```python
from build123d import *

# Parameters (mm, degrees)
F0_R     = 7.5
F0_R_2   = 6
F1_DEPTH = 2
F2_R     = 0.5


# Not quite as in the source:
# - the program builds the solid bodies; features that only make, move or delete a surface that nothing else refers to are left out


with BuildPart() as f1:
    # F0 (on Front) → F1 (new body)
    with BuildSketch(Plane.XZ):
        with Locations((0, 92.6766253437)):
            Circle(F0_R)
        with Locations((0, 92.6766253437)):
            Circle(F0_R_2, mode=Mode.SUBTRACT)
    extrude(amount=F1_DEPTH)

    # F2
    f2_edges = [f1.edges().sort_by_distance(p)[0] for p in [
        (-7.5, -2, 92.676625),
        (-6, -2, 92.676625),
        (-7.5, 0, 92.676625),
        (-6, 0, 92.676625),
    ]]
    fillet(f2_edges, radius=F2_R)


solid = f1.part
```
Work out the finished part from the listing and answer in its coordinate system (mm). Give positions to 0.01 mm unless a question says otherwise; leave off trailing zeros. Loops run counter-clockwise (first coordinate to the right, second up) from the corner with the lowest first, then second, coordinate; pieces in that order, holes last. Notation, with made-up numbers: (81.5, 6.25) -> (89.5, 6.25) arc R21 cw to (89.5, 25.25) -> close; hole circle Ø2 at (31.5, 22.25). An arc over 180 degrees is marked (long way). Put each result on its own line as item: value. Start each with the question number.
Item 1: The part is cut by section A-A (x = 0). Give the vertices of the cut face in (y, z).
Item 2: The part is cut by section B-B (y = -1.75). Give the vertices of the cut face in (x, z), then the cut area to 3 significant figures.
Item 3: The mould has two halves that part along X. Classify faces 1 (the face through (5, -2, 88)), 2 (the face through (3.226, -0.993, 97.736)), 3 (the face through (3.461, -0.993, 86.023)): released by +X, released by -X, zero draft, split by the parting line, or undercut.
Item 4: Find the intervals of material crossed by L1, parallel to Z at x = 0, y = -1.1; L2, parallel to X at y = -1.8, z = 94.75; L3, parallel to Z at x = 5.25, y = -1.4, in increasing order. Write a range as [from, to].
Item 5: Each of these flat-tipped pins is pushed along its axis until it touches: P1, Ø1, axis at x = -1.5, y = -1, coming from the +Z side; P2, Ø1, axis at y = -0.5, z = 98.5, coming from the +X side; P3, Ø1, axis at x = -5, y = -0.5, coming from the -Z side. Where does it stop, or does it pass through?
Answers below:
1. outline: (-2, 85.68) arc R0.5 ccw to (-1.5, 85.18) -> (-0.5, 85.18) arc R0.5 ccw to (0, 85.68) -> (0, 86.18) arc R0.5 ccw to (-0.5, 86.68) -> (-1.5, 86.68) arc R0.5 ccw to (-2, 86.18) -> close; (-2, 99.18) arc R0.5 ccw to (-1.5, 98.68) -> (-0.5, 98.68) arc R0.5 ccw to (0, 99.18) -> (0, 99.68) arc R0.5 ccw to (-0.5, 100.18) -> (-1.5, 100.18) arc R0.5 ccw to (-2, 99.68) -> close
2. outline: circle Ø14.87 at (0, 92.68); hole circle Ø12.13 at (0, 92.68)
2. area: 57.9 mm2
3. face 1: zero draft
3. face 2: undercut
3. face 3: split by the parting line
4. L1: [85.18, 86.68], [98.68, 100.18]
4. L2: [-7.1, -5.74], [5.74, 7.1]
4. L3: [87.32, 89.77], [95.58, 98.03]
5. P1: z = 100.11
5. P2: x = 5.28
5. P3: z = 86.68
